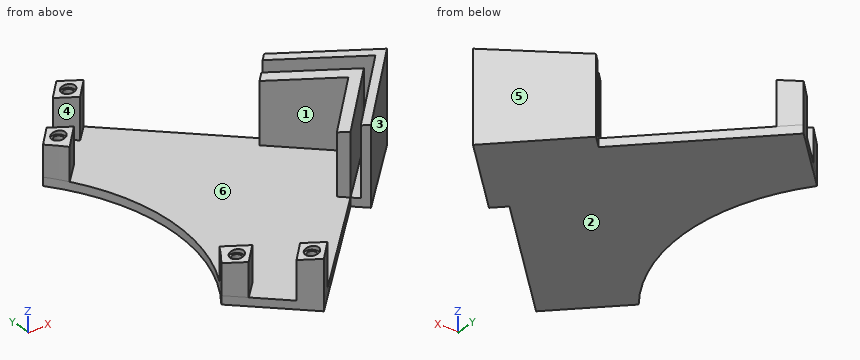
```python
from build123d import *

# Parameters (mm, degrees)
CLOSED_BOTTOM_PLATE_3MM_DEPTH       = 3
FOOT1_CURVED_R70P71_DEPTH           = 33
FOOT2_CURVED_R70P71_DEPTH           = 33
PAD4_C_BLANK_DEPTH                  = 33
PAD5_A_BLANK_DEPTH                  = 33
SLOT_BACKING_INSIDE_NORTH_DEPTH     = 35
SLOT_BACKING_INSIDE_EAST_DEPTH      = 35
TOP_OUTER_PLANE_DEPTH               = 159.981130956
TOP_OUTER_PLANE_DEPTH_BACK          = 159.981130956
SLOT_BASE_NORTH_DEPTH               = 3
SLOT_BASE_EAST_DEPTH                = 3
SLOT_OUTER_NORTH_DEPTH              = 35
SLOT_OUTER_EAST_DEPTH               = 35
CUT_EXTRUDE_2_DEPTH                 = 167.574307743
CUT_EXTRUDE_2_DEPTH_BACK            = 167.574307743
LOCATOR_1_SOCKET_D3P3_START         = 9.968990399
LOCATOR_1_SOCKET_D3P3_SKETCH_R      = 1.65
LOCATOR_1_SOCKET_D3P3_DEPTH         = 7
LOCATOR_1_ROOT_RELIEF_D4P8_START    = 13.968990399
LOCATOR_1_ROOT_RELIEF_D4P8_SKETCH_R = 2.4
LOCATOR_1_ROOT_RELIEF_D4P8_DEPTH    = 3
LOCATOR_2_SOCKET_D3P3_START         = 9.968990399
LOCATOR_2_SOCKET_D3P3_SKETCH_R      = 1.65
LOCATOR_2_SOCKET_D3P3_DEPTH         = 7
LOCATOR_2_ROOT_RELIEF_D4P8_START    = 13.968990399
LOCATOR_2_ROOT_RELIEF_D4P8_SKETCH_R = 2.4
LOCATOR_2_ROOT_RELIEF_D4P8_DEPTH    = 3
LOCATOR_3_SOCKET_D3P3_START         = 12.718990399
LOCATOR_3_SOCKET_D3P3_SKETCH_R      = 1.65
LOCATOR_3_SOCKET_D3P3_DEPTH         = 7
LOCATOR_3_ROOT_RELIEF_D4P8_START    = 16.718990399
LOCATOR_3_ROOT_RELIEF_D4P8_SKETCH_R = 2.4
LOCATOR_3_ROOT_RELIEF_D4P8_DEPTH    = 3
LOCATOR_4_SOCKET_D3P3_START         = 12.718990399
LOCATOR_4_SOCKET_D3P3_SKETCH_R      = 1.65
LOCATOR_4_SOCKET_D3P3_DEPTH         = 7
LOCATOR_4_ROOT_RELIEF_D4P8_START    = 16.718990399
LOCATOR_4_ROOT_RELIEF_D4P8_SKETCH_R = 2.4
LOCATOR_4_ROOT_RELIEF_D4P8_DEPTH    = 3


with BuildPart() as part:
    # Closed_bottom_plate_3mm_sketch → Closed_bottom_plate_3mm (new body)
    with BuildSketch(Plane.XY):
        with BuildLine():
            Line((77.781745931, -63.639610307), (141.421356237, 0))
            Line((141.421356237, 0), (77.781745931, 63.639610307))
            Line((77.781745931, 63.639610307), (56.568542495, 42.426406871))
            ThreePointArc((56.568542495, 42.426406871), (70.710678119, 0), (56.568542495, -42.426406871))
            Line((56.568542495, -42.426406871), (77.781745931, -63.639610307))
        make_face()
    extrude(amount=CLOSED_BOTTOM_PLATE_3MM_DEPTH)

    # Foot1_curved_R70p71_sketch → Foot1_curved_R70p71 (add)
    with BuildSketch(Plane.XY):
        with BuildLine():
            Line((62.225396744, 48.083261121), (67.882250994, 42.426406871))
            Line((67.882250994, 42.426406871), (61.080791676, 35.624947554))
            ThreePointArc((61.080791676, 35.624947554), (58.922885367, 39.090837546), (56.568542495, 42.426406871))
            Line((56.568542495, 42.426406871), (62.225396744, 48.083261121))
        make_face()
    extrude(amount=FOOT1_CURVED_R70P71_DEPTH)

    # Foot2_curved_R70p71_sketch → Foot2_curved_R70p71 (add)
    with BuildSketch(Plane.XY):
        with BuildLine():
            Line((62.225396744, -48.083261121), (67.882250994, -42.426406871))
            Line((67.882250994, -42.426406871), (61.080791676, -35.624947554))
            ThreePointArc((61.080791676, -35.624947554), (58.922885367, -39.090837546), (56.568542495, -42.426406871))
            Line((56.568542495, -42.426406871), (62.225396744, -48.083261121))
        make_face()
    extrude(amount=FOOT2_CURVED_R70P71_DEPTH)

    # Pad4_C_blank_sketch → Pad4_C_blank (add)
    with BuildSketch(Plane.XY):
        Polygon((72.124891681, 57.982756057), (77.781745931, 52.325901808), (83.43860018, 57.982756057), (77.781745931, 63.639610307), align=None)
    extrude(amount=PAD4_C_BLANK_DEPTH)

    # Pad5_A_blank_sketch → Pad5_A_blank (add)
    with BuildSketch(Plane.XY):
        Polygon((72.124891681, -57.982756057), (77.781745931, -63.639610307), (83.43860018, -57.982756057), (77.781745931, -52.325901808), align=None)
    extrude(amount=PAD5_A_BLANK_DEPTH)

    # Slot_backing_inside_north_sketch → Slot_backing_inside_north (add)
    with BuildSketch(Plane.XY):
        Polygon((117.379725677, 18.384776311), (138.592929113, -2.828427125), (141.421356237, 0), (120.208152802, 21.213203436), align=None)
    extrude(amount=SLOT_BACKING_INSIDE_NORTH_DEPTH)

    # Slot_backing_inside_east_sketch → Slot_backing_inside_east (add)
    with BuildSketch(Plane.XY):
        Polygon((117.379725677, -18.384776311), (120.208152802, -21.213203436), (141.421356237, 0), (138.592929113, 2.828427125), align=None)
    extrude(amount=SLOT_BACKING_INSIDE_EAST_DEPTH)

    # Top_outer_plane_sketch → Top_outer_plane (cut, two sides: drawn at the far end of the back side and taken through both)
    with BuildSketch(Plane(origin=(0, 0, 0), x_dir=(1, 0, 0), z_dir=(0, 1, 0)).offset(-TOP_OUTER_PLANE_DEPTH_BACK)):
        Polygon((-100, 13.708679131), (250, -48.163164223), (250, -100), (-100, -100), align=None)
    extrude(amount=TOP_OUTER_PLANE_DEPTH + TOP_OUTER_PLANE_DEPTH_BACK, mode=Mode.SUBTRACT)

    # Slot_base_north_sketch → Slot_base_north (add)
    with BuildSketch(Plane.XY):
        Polygon((117.379725677, 18.384776311), (142.8355698, -7.071067812), (149.906637612, 0), (124.450793489, 25.455844123), align=None)
    extrude(amount=SLOT_BASE_NORTH_DEPTH)

    # Slot_base_east_sketch → Slot_base_east (add)
    with BuildSketch(Plane.XY):
        Polygon((117.379725677, -18.384776311), (124.450793489, -25.455844123), (149.906637612, 0), (142.8355698, 7.071067812), align=None)
    extrude(amount=SLOT_BASE_EAST_DEPTH)

    # Slot_outer_north_sketch → Slot_outer_north (add)
    with BuildSketch(Plane.XY):
        Polygon((122.329473145, 23.334523779), (147.785317268, -2.121320344), (149.906637612, 0), (124.450793489, 25.455844123), align=None)
    extrude(amount=SLOT_OUTER_NORTH_DEPTH)

    # Slot_outer_east_sketch → Slot_outer_east (add)
    with BuildSketch(Plane.XY):
        Polygon((122.329473145, -23.334523779), (124.450793489, -25.455844123), (149.906637612, 0), (147.785317268, 2.121320344), align=None)
    extrude(amount=SLOT_OUTER_EAST_DEPTH)

    # 草图13 → 切除-拉伸2 (cut, two sides: drawn at the far end of the back side and taken through both)
    with BuildSketch(Plane(origin=(0, 0, 0), x_dir=(1, 0, 0), z_dir=(0, 1, 0)).offset(-CUT_EXTRUDE_2_DEPTH_BACK)):
        Polygon((-100, 11.67766953), (250, -50.194173824), (250, -100), (-100, -100), align=None)
    extrude(amount=CUT_EXTRUDE_2_DEPTH + CUT_EXTRUDE_2_DEPTH_BACK, mode=Mode.SUBTRACT)

    # Locator_1_socket_D3p3_sketch → Locator_1_socket_D3p3 (cut)
    with BuildSketch(Plane.XY.offset(LOCATOR_1_SOCKET_D3P3_START)):
        with Locations(Location((62.225396744, 42.426406871, 0), (0, 0, 180))):
            Circle(LOCATOR_1_SOCKET_D3P3_SKETCH_R)
    extrude(amount=LOCATOR_1_SOCKET_D3P3_DEPTH, mode=Mode.SUBTRACT)

    # Locator_1_root_relief_D4p8_sketch → Locator_1_root_relief_D4p8 (cut)
    with BuildSketch(Plane.XY.offset(LOCATOR_1_ROOT_RELIEF_D4P8_START)):
        with Locations(Location((62.225396744, 42.426406871, 0), (0, 0, 180))):
            Circle(LOCATOR_1_ROOT_RELIEF_D4P8_SKETCH_R)
    extrude(amount=LOCATOR_1_ROOT_RELIEF_D4P8_DEPTH, mode=Mode.SUBTRACT)

    # Locator_2_socket_D3p3_sketch → Locator_2_socket_D3p3 (cut)
    with BuildSketch(Plane.XY.offset(LOCATOR_2_SOCKET_D3P3_START)):
        with Locations(Location((62.225396744, -42.426406871, 0), (0, 0, 180))):
            Circle(LOCATOR_2_SOCKET_D3P3_SKETCH_R)
    extrude(amount=LOCATOR_2_SOCKET_D3P3_DEPTH, mode=Mode.SUBTRACT)

    # Locator_2_root_relief_D4p8_sketch → Locator_2_root_relief_D4p8 (cut)
    with BuildSketch(Plane.XY.offset(LOCATOR_2_ROOT_RELIEF_D4P8_START)):
        with Locations(Location((62.225396744, -42.426406871, 0), (0, 0, 180))):
            Circle(LOCATOR_2_ROOT_RELIEF_D4P8_SKETCH_R)
    extrude(amount=LOCATOR_2_ROOT_RELIEF_D4P8_DEPTH, mode=Mode.SUBTRACT)

    # Locator_3_socket_D3p3_sketch → Locator_3_socket_D3p3 (cut)
    with BuildSketch(Plane.XY.offset(LOCATOR_3_SOCKET_D3P3_START)):
        with Locations(Location((77.781745931, 57.982756057, 0), (0, 0, 180))):
            Circle(LOCATOR_3_SOCKET_D3P3_SKETCH_R)
    extrude(amount=LOCATOR_3_SOCKET_D3P3_DEPTH, mode=Mode.SUBTRACT)

    # Locator_3_root_relief_D4p8_sketch → Locator_3_root_relief_D4p8 (cut)
    with BuildSketch(Plane.XY.offset(LOCATOR_3_ROOT_RELIEF_D4P8_START)):
        with Locations(Location((77.781745931, 57.982756057, 0), (0, 0, 180))):
            Circle(LOCATOR_3_ROOT_RELIEF_D4P8_SKETCH_R)
    extrude(amount=LOCATOR_3_ROOT_RELIEF_D4P8_DEPTH, mode=Mode.SUBTRACT)

    # Locator_4_socket_D3p3_sketch → Locator_4_socket_D3p3 (cut)
    with BuildSketch(Plane.XY.offset(LOCATOR_4_SOCKET_D3P3_START)):
        with Locations(Location((77.781745931, -57.982756057, 0), (0, 0, 180))):
            Circle(LOCATOR_4_SOCKET_D3P3_SKETCH_R)
    extrude(amount=LOCATOR_4_SOCKET_D3P3_DEPTH, mode=Mode.SUBTRACT)

    # Locator_4_root_relief_D4p8_sketch → Locator_4_root_relief_D4p8 (cut)
    with BuildSketch(Plane.XY.offset(LOCATOR_4_ROOT_RELIEF_D4P8_START)):
        with Locations(Location((77.781745931, -57.982756057, 0), (0, 0, 180))):
            Circle(LOCATOR_4_ROOT_RELIEF_D4P8_SKETCH_R)
    extrude(amount=LOCATOR_4_ROOT_RELIEF_D4P8_DEPTH, mode=Mode.SUBTRACT)


solid = part.part
```
Verification items for the finished model (mm, model axes). Face numbers are marked on the shaded views. A direction names the side the tool comes from. Coordinates: 2 decimals unless noted, no trailing zeros. Write each loop counter-clockwise with the first axis right and the second up, starting at its lowest first coordinate (ties: lowest second). Pieces come first, ordered by that corner, then holes. Notation, with made-up numbers: (-39, 74) - (-32, 74) arc R20 ccw to (-32, 92) - close; hole circle Ø7 at (-31.75, 26). An arc over 180 degrees is marked (long way). One line per question, with ' | ' between items. Start each with the question number.
1. Section check D-D (x = 81.5). Enter the section's corners in (y, z), plus the area to 3 significant figures.
2. Section check A-A (z = 23). Enter the section's corners in (x, y), plus the area to 3 significant figures.
3. Access from +Z, -Z, +X, -X, +Y, -Y to the whole of each face (thin tool, end or side, straight path). Record for the marked faces 4, 5 and 6.
4. Section check C-C (y = 8.5). Enter the section's corners in (x, z).
5. Gauge pin test, flat ends, axial feed: P1, Ø3, axis at x = 80, z = 15.5, coming from the -Y side; P2, Ø1, axis at x = 78.5, y = -58.5, coming from the +Z side; P3, Ø2.5, axis at x = 78, y = -59, coming from the +Z side. Record the tip position at first contact, or that the pin passes through.
6. Draft check along Y on the marked faces 1, 2 and 3. Enter one of: released by +Y, released by -Y, zero draft, split by the parting line, or undercut.
7. Section check B-B (z = 7). Enter the section's corners in (x, y), plus the area to 3 significant figures.
8. Material ranges on line 1 along Y through (x, z) = (123, 11.5); line 2 along Y through (x, z) = (65.5, 13); line 3 along Z through (x, y) = (61, -39), recorded low to high.
Computed values:
1) outline: (-59.92, 0) - (59.92, 0) - (59.92, 18.38) - (56.04, 18.38) - (56.04, 3) - (-56.04, 3) - (-56.04, 18.38) - (-59.92, 18.38) - close | area: 479 mm²
2) outline: (117.38, -18.38) - (120.21, -21.21) - (141.42, 0) - (120.21, 21.21) - (117.38, 18.38) - (135.76, 0) - close; (122.33, -23.33) - (124.45, -25.46) - (149.91, 0) - (124.45, 25.46) - (122.33, 23.33) - (145.66, 0) - close | area: 431 mm²
3) face 4: +Z, -X | face 5: +Z, -Z, +X, +Y | face 6: +Z
4) outline: (70.2, 0) - (141.41, 0) - (141.41, 31) - (137.16, 30.25) - (137.16, 3) - (132.92, 3) - (132.92, 27.47) - (127.26, 26.47) - (127.26, 3) - (70.2, 3) - close
5) P1: y = -62.92 | P2: z = 12.72 | P3: z = 16.72
6) face 1: undercut | face 2: zero draft | face 3: released by -Y
7) outline: (56.57, -42.43) - (62.23, -48.08) - (67.88, -42.43) - (61.08, -35.62) arc R70.71 cw to start; (56.57, 42.43) arc R70.71 cw to (61.08, 35.62) - (67.88, 42.43) - (62.23, 48.08) - close; (72.12, -57.98) - (77.78, -63.64) - (83.44, -57.98) - (77.78, -52.33) - close; (72.12, 57.98) - (77.78, 52.33) - (83.44, 57.98) - (77.78, 63.64) - close; (117.38, -18.38) - (120.21, -21.21) - (141.42, 0) - (120.21, 21.21) - (117.38, 18.38) - (135.76, 0) - close; (122.33, -23.33) - (124.45, -25.46) - (149.91, 0) - (124.45, 25.46) - (122.33, 23.33) - (145.66, 0) - close | area: 699 mm²
8) line 1: -24.01 to -22.66, -18.42 to -12.76, 12.76 to 18.42, 22.66 to 24.01 | line 2: -44.81 to -40.04, 40.04 to 44.81 | line 3: 0 to 14.75
